For this review, take the finished solid that the model builds, in its own axes (mm). Round coordinates to 2 decimals unless told otherwise and drop trailing zeros. Order: outer loops, then holes, each group sorted by start corner. A loop starts at its lowest first (then second) coordinate and runs counter-clockwise, first axis right, second up. Notation, with made-up numbers: M 6.5,28 L 55.5,28 A22 ccw 55.5,48 Z; hole C 41,87 d7. An arc over 180 degrees is marked long. Put each result on its own line as item: value.
from build123d import *

# Parameters (mm, degrees)
F0_R     = 127
F1_DEPTH = 4.7625
F2_W     = 12.7
F2_H     = 76.2
F3_DEPTH = 25.4
F4_SIZE  = 5.08
F5_R     = 6.35
F6_DEPTH = 4.7635
F7_W     = 3.175
F7_H     = 127
F8_DEPTH = 4.7635


with BuildPart() as f1:
    # F0 (on Front) → F1 (new body)
    with BuildSketch(Plane.XZ):
        Circle(F0_R)
    extrude(amount=F1_DEPTH)

    # F5 (on face) → F6 (cut, through all)
    with BuildSketch(Plane.XZ.offset(4.7625)):
        with Locations((9.505124, 61.177523)):
            Circle(F5_R)
        with Locations((9.505124, 40.313245)):
            Circle(F5_R)
    extrude(amount=-F6_DEPTH, mode=Mode.SUBTRACT)

    # F7 (on face) → F8 (cut, through all)
    with BuildSketch(Plane.XZ.offset(4.7625)):
        with Locations((24.478537, 48.747311)):
            Rectangle(F7_W, F7_H)
    extrude(amount=-F8_DEPTH, mode=Mode.SUBTRACT)


with BuildPart() as f3:
    # F2 (on face) → F3 (new body)
    with BuildSketch(Plane.XZ.offset(4.7625)):
        with Locations((-221.724585, -33.983209)):
            Rectangle(F2_W, F2_H)
    extrude(amount=F3_DEPTH)

    # F4
    f4_edges = [f3.edges().sort_by_distance(p)[0] for p in [
        (-228.074585, -30.1625, -33.983209),
        (-215.374585, -30.1625, -33.983209),
        (-221.724585, -30.1625, 4.116791),
        (-221.724585, -30.1625, -72.083209),
    ]]
    chamfer(f4_edges, length=F4_SIZE)


solid = f1.part
(1) Add section B-B on z = 105. Give the boundary of the cut face in (x, y).
A:
outline: M -71.44,-4.76 L 22.89,-4.76 L 22.89,0 L -71.44,0 Z; M 26.07,-4.76 L 71.44,-4.76 L 71.44,0 L 26.07,0 Z
(2) Add section A-A on x = 9. Give the boundary of the cut face in (y, z), then the cut area to 3 significant figures.
A:
outline: M -4.76,-126.68 L 0,-126.68 L 0,33.98 L -4.76,33.98 Z; M -4.76,46.64 L 0,46.64 L 0,54.85 L -4.76,54.85 Z; M -4.76,67.51 L 0,67.51 L 0,126.68 L -4.76,126.68 Z
area: 1,090 mm2
(3) To check wall thickness, follow L1, parallel to X at y = -1.65, z = 42; L2, parallel to X at y = -0.55, z = 40.5; L3, parallel to Z at x = 26, y = -0.8. State the ranges of each line that lie inside material, in increasing order.
A:
L1: x = -119.85 to 3.38, 15.63 to 22.89, 26.07 to 119.85
L2: x = -120.37 to 3.16, 15.85 to 22.89, 26.07 to 120.37
L3: z = -124.31 to -14.75, 112.25 to 124.31
(4) Add section D-D on z = -74. Give the boundary of the cut face in (x, y).
A:
outline: M -103.21,-4.76 L 103.21,-4.76 L 103.21,0 L -103.21,0 Z
(5) Draft analysis for pull direction X (two halves, no side actions). For faces 1 (the face through (-27.53, -2.35, -123.98)), 2 (the face through (-2, -4.762, 2)), 3 (the face through (8.678, -2.415, 67.473)), state which applies: released by +X, released by -X, zero draft, split by the parting line, or undercut.
A:
face 1: split by the parting line
face 2: zero draft
face 3: undercut
(6) Add section C-C on y = -3.1. Give the boundary of the cut face in (x, z), then the cut area to 3 significant figures.
A:
outline: C 0,0 d254; hole C 9.51,40.31 d12.7; hole C 9.51,61.18 d12.7; hole M 22.89,-14.75 L 26.07,-14.75 L 26.07,112.25 L 22.89,112.25 Z
area: 50,000 mm2
(7) Insertion check: pin 1 Ø2.5 at (x, y) = (25, -3) entering from -Z; pin 2 Ø2 at (y, z) = (-0.5, 22) entering from +X. Each pin has a flat end and moves straight along its axis. Give the tip position at first contact, or say it passes through.
A:
pin 1: stops at z = -124.76
pin 2: stops at x = 125.25
